Source: CAD feature listing. Evaluate the final solid. Frame: model axes, mm. A direction names the side the tool comes from. Coordinates: 2 decimals unless noted, no trailing zeros. Order: outer loops, then holes, each group sorted by start corner. A loop starts at its lowest first (then second) coordinate and runs counter-clockwise, first axis right, second up. Notation, with made-up numbers: (43, 53) - (49, 53) arc R20 cw to (49, 81) - close; hole circle Ø2 at (73.5, 68). An arc over 180 degrees is marked (long way). One line per question, with ' | ' between items. Start each with the question number.
(1) Draft query along Y for faces 4 (the flat face through (1, 1, -4.762)), 5 (the flat face through (0, 0, 0)), 6 (the flat face through (-0.783, 1.381, -0.067)). Return one class per face: +Y half, -Y half, draft (parallel to the pull), parting line (faces both ways), or undercut.
(2) Access query for faces 1 (the flat face through (0, 0, 4.189)), 2 (the flat face through (0.8, 1.37, -0.07)), 3 (the cylindrical face through (0.87, 0.19, -2.28)). Directions: +Z, -Z, +X, -X, +Y, -Y. A direction counts if a zero-diameter tool reaches every point of the face in a straight line with its end or side. Return the directions, or none.
(3) Contact query for flat-ended pins moving along their axis: P1, Ø1.5, axis at x = 0, y = 0, coming from the -Z side; P2, Ø0.6, axis at x = 0, y = 0.5, coming from the +Z side; P3, Ø1.4, axis at x = 0.5, y = -0.5, coming from the -Z side. Output: stop coordinate, or through.
(4) Section A-A (z = -3.75). Return the cut outline in (x, y).
(5) Section B-B (z = 4). Return the cut outline in (x, y), then the cut area to 3 significant figures.
(6) Line query: line 1 along X through (y, z) = (0, -1.1); line 2 along Z through (x, y) = (-0.8, -0.8); line 3 along Y through (x, z) = (0.35, -2.5). Output: solid intervals per line, ascending.
Autodesk Fusion 360 part; units mm, degrees
sketch "Sketch1" plane through (0, 0, 0) normal (0, 0, 1) x (1, 0, 0)
  line L0 (1.5875, 0.9165) -> (0, 1.8331)
  line L1 (0, 1.8331) -> (-1.5875, 0.9165)
  line L2 (-1.5875, 0.9165) -> (-1.5875, -0.9165)
  line L3 (-1.5875, -0.9165) -> (0, -1.8331)
  line L4 (0, -1.8331) -> (1.5875, -0.9165)
  line L5 (1.5875, -0.9165) -> (1.5875, 0.9165)
  circle A0 centre (0, 0) radius 1.5875 construction
  dimension "d4" = 3.175
extrude "Extrude1" add sketch "Sketch1" along normal mid plane 9.525
sketch "Sketch2" plane through (0, 0, 0) normal (1, 0, 0) x (0, 1, 0)
  line L0 (1.8331, 4.7625) -> (-1.8331, 4.7625)
  line L1 (-1.8331, -4.7625) -> (1.8331, -4.7625)
  line L2 (-1.5875, 0) -> (-1.5875, 4.7625) construction
  line L3 (-1.5875, 0) -> (-1.5875, -4.7625) construction
  line L4 (-1.8331, 4.7625) -> (-1.8331, 4.6207)
  line L5 (-1.8331, 4.6207) -> (-1.5875, 4.7625)
  line L6 (-1.5875, 0) -> (0, 0) construction
  line L7 (0, 0) -> (0, 4.7625)
  line L8 (-1.8331, -4.6207) -> (-1.5875, -4.7625)
  line L9 (-1.8331, -4.7625) -> (-1.8331, -4.6207)
  point P0 (-1.5875, 0)
  point P1 (1.5875, 0)
  dimension "d7" = 30
revolve "Revolve1" cut sketch "Sketch2" angle 360 about axis through (0, 0, 0) along (0, 0, 1)
sketch "Sketch3" plane through (0, 0, 0) normal (0, 1, 0) x (1, 0, 0)
  line L0 (-1.5875, -4.7625) -> (1.5875, -4.7625)
  line L1 (1.5875, 4.7625) -> (-1.5875, 4.7625)
  line L2 (0, -4.7625) -> (0, 4.7625)
  line L3 (0, -4.1891) -> (0.5734, -4.1891)
  line L4 (0.5734, -4.1891) -> (1.1468, -4.7625)
  line L5 (0, 0) -> (1.5875, 0) construction
  line L6 (0, 4.1891) -> (0.5734, 4.1891)
  line L7 (0.5734, 4.1891) -> (1.1468, 4.7625)
  dimension "d9" = 45
  dimension "d10" = 2.2936
  dimension "d11" = 1.1468
sketch "Sketch4" plane through (0, 0, 4.7625) normal (0, 0, 1) x (-1, 0, 0)
  arc A0 (-0.7937, -1.3748) -> (0.7937, -1.3748) centre (0, 0) ccw
  arc A1 (0.7937, -1.3748) -> (1.5875, 0) centre (0, 0) ccw
  arc A2 (1.5875, 0) -> (0.7937, 1.3748) centre (0, 0) ccw
  arc A3 (0.7937, 1.3748) -> (-0.7937, 1.3748) centre (0, 0) ccw
  arc A4 (-0.7937, 1.3748) -> (-1.5875, 0) centre (0, 0) ccw
  arc A5 (-1.5875, 0) -> (-0.7937, -1.3748) centre (0, 0) ccw
hole "Hole1" at (0, 0, 0) direction (0, 0, -1) diameter 1.778 end through all
revolve "Revolve2" cut sketch "Sketch3" angle 360 about axis through (0, 0, 4.7625) along (0, 0, -1)
equation "Length = ( 3 / 8 ) * 1 in"
equation "HexWidth = ( 1 / 8 ) * 1 in"
equation "MajorDia = 0.086 in"
equation "d4 = HexWidth"
equation "d5 = Length"
equation "d10 = MajorDia * 1.05"
equation "d11 = d10 / 2"
properties part number "91780A028"
Response values:
1) face 4: draft | face 5: undercut | face 6: +Y half
2) face 1: +Z | face 2: +Z, -Z, +X, +Y | face 3: -Z
3) P1: stops at z = 0 | P2: stops at z = 4.42 | P3: stops at z = -4.76
4) outline: (-1.59, -0.92) - (0, -1.83) - (1.59, -0.92) - (1.59, 0.92) - (0, 1.83) - (-1.59, 0.92) - close; hole circle Ø1.78 at (0, 0)
5) outline: (-1.59, -0.92) - (0, -1.83) - (1.59, -0.92) - (1.59, 0.92) - (0, 1.83) - (-1.59, 0.92) - close | area: 8.73 mm²
6) line 1: x = -1.59 to -0.89, 0.89 to 1.59 | line 2: z = -4.75 to 4.75 | line 3: y = -1.63 to -0.82, 0.82 to 1.63
